Verification items for the finished model (mm, model axes). A direction names the side the tool comes from. Coordinates: 2 decimals unless noted, no trailing zeros. Order: outer loops, then holes, each group sorted by start corner. A loop starts at its lowest first (then second) coordinate and runs counter-clockwise, first axis right, second up. Notation, with made-up numbers: (65.5, -24.5) -> (87.5, -24.5) arc R7 ccw to (87.5, -13.5) -> close; hole circle Ø2 at (-17.75, 65.25). An arc over 180 degrees is marked (long way). Write item = value, one per line. Start each with the question number.
1. Cross-section at D-D on z = -17. Record the cut outline in (x, y).
2. Cross-section at B-B on x = 8.5. Record the cut outline in (y, z).
3. Cross-section at C-C on y = -6. Record the cut outline in (x, z), plus the area to 3 significant figures.
4. Release check for a two-part mould opening along Y. For faces 4 (the cylindrical face through (-67, 0, -33)), 5 (the flat face through (-1, -8, 0)), 6 (the flat face through (67, 1, 0)) record: +Y half, -Y half, draft (parallel to the pull), parting line (faces both ways), or undercut.
5. Go/stop test with flat-tipped pins: P1, Ø0.6, axis at y = 0.5, z = -1.5, coming from the +X side; P2, Ø4, axis at y = 1, z = 16.5, coming from the +X side; P3, Ø2.5, axis at x = 62.5, y = -1, coming from the -Z side; P4, Ø3, axis at y = 6, z = 18, coming from the -X side. Record where each tip stops, or that it passes through.
6. Set-up check for faces 1 (the flat face through (67, -1, 0)), 2 (the cylindrical face through (0.87, 5.93, -32.82)), 3 (the flat face through (46, 1.27, -31)): record each of +Z, -Z, +X, -X, +Y, -Y from which the full face is reachable in a straight line by a thin tool's end or side.
7. Cross-section at A-A on z = 0. Record the cut outline in (x, y), plus the area to 3 significant figures.
8. Thickness scan on line 1 along Y through (x, z) = (58.84, 34.45); line 2 along Z through (x, y) = (55, -1); line 3 along X through (y, z) = (0.25, -28.5). Record the ranges inside material, lowest first. Write a range as from..to.
from build123d import *

# Parameters (mm, degrees)
SKETCH1_W                  = 138.5
SKETCH1_H                  = 70
BOSS_EXTRUDE1_DEPTH        = 8
FILLET1_R                  = 7.25
SKETCH3_W                  = 12.7
SKETCH3_H                  = 5.08
USB_A_DEPTH                = 11.25
SKETCH4_W                  = 7
SKETCH4_H                  = 2
USB_MICRO_NOTTOSCALE_DEPTH = 5
SKETCH5_W                  = 8.382
SKETCH5_H                  = 2.54
USB_C_DEPTH                = 8
FILLET2_R                  = 1.27
SKETCH6_W                  = 6.9
SKETCH6_H                  = 3.5
BATTERY_LEVEL_DEPTH        = 0.5
FILLET3_R                  = 1.75
SKETCH7_R                  = 0.3
BATTERY_LIGHTS_DEPTH       = 1


# Some blends are built 0.0001 mm under size
with BuildPart() as part:
    # Sketch1 → Boss-Extrude1 (new, symmetric)
    with BuildSketch(Plane(origin=(0, 0, 0), x_dir=(1, 0, 0), z_dir=(0, 1, 0))):
        Rectangle(SKETCH1_W, SKETCH1_H)
    extrude(amount=BOSS_EXTRUDE1_DEPTH, both=True)

    # Fillet1
    fillet1_edges = [part.edges().sort_by_distance(p)[0] for p in [
        (-69.25, 8, 0),
        (0, 8, 35),
        (69.25, 8, 0),
        (0, -8, 35),
        (-69.25, -8, 0),
        (0, -8, -35),
        (69.25, -8, 0),
        (69.25, 0, 35),
        (-69.25, 0, 35),
        (-69.25, 0, -35),
        (69.25, 0, -35),
        (0, 8, -35),
    ]]
    fillet(fillet1_edges, radius=FILLET1_R)

    # Sketch3 → USB-A (cut)
    with BuildSketch(Plane(origin=(69.25, 0, 0), x_dir=(0, 0, -1), z_dir=(1, 0, 0))):
        with Locations((-19.15, 0)):
            Rectangle(SKETCH3_W, SKETCH3_H)
        with Locations((19.15, 0)):
            Rectangle(SKETCH3_W, SKETCH3_H)
    extrude(amount=-USB_A_DEPTH, mode=Mode.SUBTRACT)

    # Sketch4 → USB-micro-NOTtoSCALE (cut)
    with BuildSketch(Plane(origin=(69.25, 0, 0), x_dir=(0, 0, -1), z_dir=(1, 0, 0))):
        Rectangle(SKETCH4_W, SKETCH4_H)
    extrude(amount=-USB_MICRO_NOTTOSCALE_DEPTH, mode=Mode.SUBTRACT)

    # Sketch5 → USB-C (cut)
    with BuildSketch(Plane(origin=(0, 0, -35), x_dir=(-1, 0, 0), z_dir=(0, 0, -1))):
        with Locations((-46.009, 0)):
            Rectangle(SKETCH5_W, SKETCH5_H)
    extrude(amount=-USB_C_DEPTH, mode=Mode.SUBTRACT)

    # Fillet2
    fillet2_edges = [part.edges().sort_by_distance(p)[0] for p in [
        (41.818, 1.27, -30.990663839),
        (41.818, -1.27, -30.990663839),
        (50.2, -1.27, -30.990663839),
        (50.2, 1.27, -30.990663839),
    ]]
    fillet(fillet2_edges, radius=FILLET2_R - 0.0001)  # a hair under: the kernel refuses the full size

    # Sketch6 → battery level (add)
    with BuildSketch(Plane.XY.offset(35)):
        with Locations((43.49, 0)):
            Rectangle(SKETCH6_W, SKETCH6_H)
    extrude(amount=BATTERY_LEVEL_DEPTH)

    # Fillet3
    # the kernel refuses this fillet: 1.75 mm, written as the material it takes off along each edge
    with BuildSketch(Plane(origin=(40.04, -1.75, 35), x_dir=(0, 1, 0), z_dir=(0, 0, 1))) as fillet3_piece_1:
        with BuildLine():
            CenterArc((FILLET3_R, -FILLET3_R), FILLET3_R, 90, 90)
            Line((0, -FILLET3_R), (0, 0))
            Line((0, 0), (FILLET3_R, 0))
        make_face()
    extrude(amount=4.875, mode=Mode.SUBTRACT)
    with BuildSketch(Plane(origin=(40.04, 1.75, 35), x_dir=(0, -1, 0), z_dir=(0, 0, 1)), Plane(origin=(46.94, -1.75, 35), x_dir=(0, 1, 0), z_dir=(0, 0, 1)), Plane(origin=(46.94, 1.75, 35), x_dir=(-1, 0, 0), z_dir=(0, 0, 1))) as fillet3_piece_2:
        with BuildLine():
            CenterArc((FILLET3_R, FILLET3_R), FILLET3_R, 180, 90)
            Line((0, FILLET3_R), (0, 0))
            Line((0, 0), (FILLET3_R, 0))
        make_face()
    extrude(amount=4.875, mode=Mode.SUBTRACT)

    # Sketch7 → battery lights (cut)
    with BuildSketch(Plane.XY.offset(35)):
        with Locations((51.94, 0)):
            Circle(SKETCH7_R)
        with Locations((54.24, 0)):
            Circle(SKETCH7_R)
        with Locations((56.54, 0)):
            Circle(SKETCH7_R)
        with Locations((58.84, 0)):
            Circle(SKETCH7_R)
    extrude(amount=-BATTERY_LIGHTS_DEPTH, mode=Mode.SUBTRACT)


solid = part.part
Worked out:
q1.outline = (-69.25, -0.75) arc R7.25 ccw to (-62, -8) -> (62, -8) arc R7.25 ccw to (69.03, -2.54) -> (58, -2.54) -> (58, 2.54) -> (69.03, 2.54) arc R7.25 ccw to (62, 8) -> (-62, 8) arc R7.25 ccw to (-69.25, 0.75) -> close
q2.outline = (-8, -27.75) arc R7.25 ccw to (-0.75, -35) -> (0.75, -35) arc R7.25 ccw to (8, -27.75) -> (8, 27.75) arc R7.25 ccw to (0.75, 35) -> (-0.75, 35) arc R7.25 ccw to (-8, 27.75) -> close
q3.outline = (-67, -27.75) arc R5 ccw to (-62, -32.75) -> (62, -32.75) arc R5 ccw to (67, -27.75) -> (67, 27.75) arc R5 ccw to (62, 32.75) -> (-62, 32.75) arc R5 ccw to (-67, 27.75) -> close
q3.area = 8,760 mm²
q4.face_4 = draft
q4.face_5 = -Y half
q4.face_6 = undercut
q5.P1 = 64.25
q5.P2 = 69.03
q5.P3 = -35
q5.P4 = -68.2
q6.face_1 = +X
q6.face_2 = -Z, +X, -X, +Y
q6.face_3 = -Z
q7.outline = (-69.25, -0.75) arc R7.25 ccw to (-62, -8) -> (62, -8) arc R7.25 ccw to (69.25, -1) -> (64.25, -1) -> (64.25, 1) -> (69.25, 1) arc R7.25 ccw to (62, 8) -> (-62, 8) arc R7.25 ccw to (-69.25, 0.75) -> close
q7.area = 2,160 mm²
q8.line_1 = -3.52..-0.3, 0.3..3.52
q8.line_2 = -35..35
q8.line_3 = -69.21..41.84, 50.18..69.21
